The drawing under review shows one solid part. Ordinate dimensions are in mm from its lowest x, y, z. A direction names the side the tool comes from. Round coordinates to 2 decimals unless told otherwise and drop trailing zeros. Write each loop counter-clockwise with the first axis right and the second up, starting at its lowest first coordinate (ties: lowest second). Pieces come first, ordered by that corner, then holes. Notation, with made-up numbers: (30.25, -18.5) -> (34.25, -18.5) arc R18 ccw to (34.25, 3.5) -> close; hole circle Ø5 at (8.25, 47.25). An arc over 180 degrees is marked (long way). Answer in a Markdown table with one row per item.
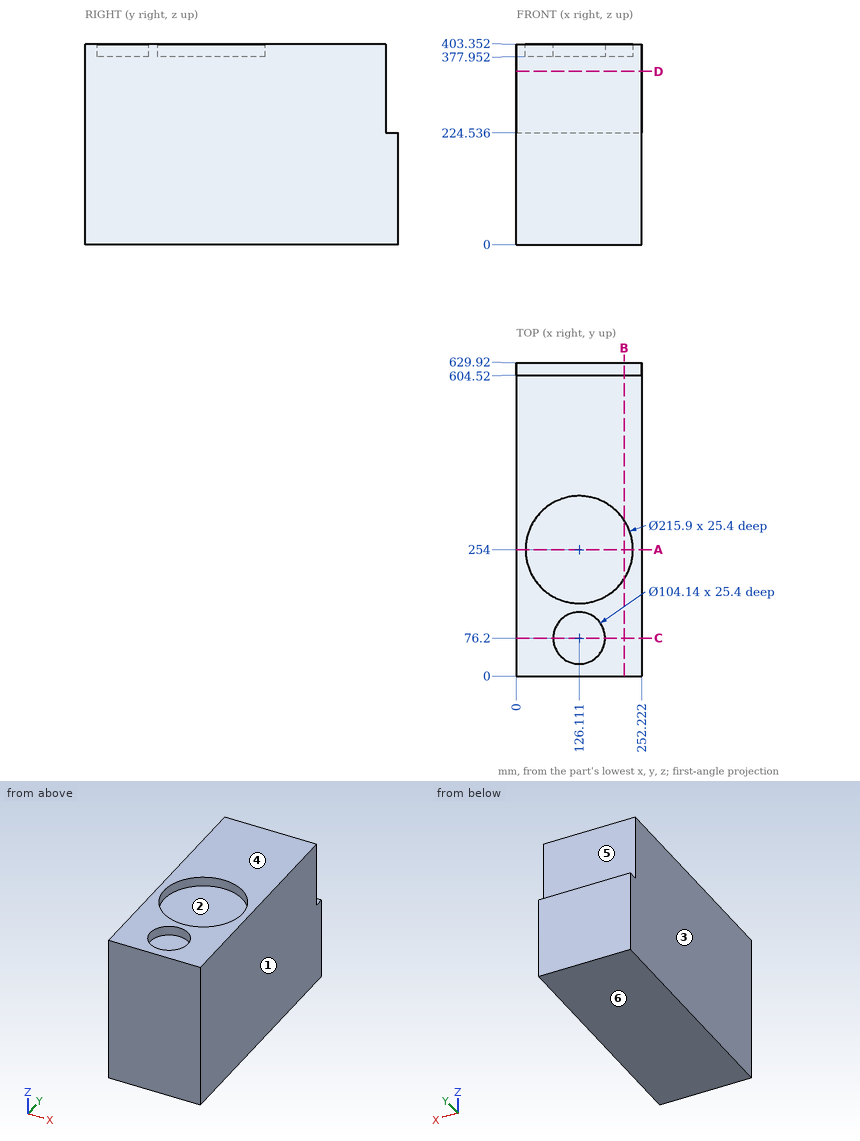
1) Consider section C-C on y = 76.2. State the section outline as (x, z) points, then the cut area to 3 significant figures.
Solved:
| item | result |
|---|---|
| outline | (0, 0) -> (252.22, 0) -> (252.22, 403.35) -> (178.18, 403.35) -> (178.18, 377.95) -> (74.04, 377.95) -> (74.04, 403.35) -> (0, 403.35) -> close |
| area | 99,100 mm² |
2) Consider section B-B on x = 216.5. State the section outline as (y, z) points, then the cut area to 3 significant figures.
Solved:
| item | result |
|---|---|
| outline | (0, 0) -> (629.92, 0) -> (629.92, 224.54) -> (604.52, 224.54) -> (604.52, 403.35) -> (313.02, 403.35) -> (313.02, 377.95) -> (194.98, 377.95) -> (194.98, 403.35) -> (0, 403.35) -> close |
| area | 247,000 mm² |
3) For the marked faces 5 and 6, list the 3-axis set-ups (+Z, -Z, +X, -X, +Y, -Y) from which the entire face can be reached by the end or side of a thin tool; tool diameter is ignored.
Solved:
| item | result |
|---|---|
| face 5 | +Z, +X, -X, +Y |
| face 6 | -Z, +X, -X, +Y, -Y |
4) Clearance check with flat-ended pins moving along their axes: pin 1 Ø1.5 at (x, y) = (111.5, 333) entering from +Z; pin 2 Ø10 at (x, z) = (146, 310) entering from +Y; pin 3 Ø12.5 at (x, y) = (127.5, 619) entering from +Z. State where each tip first meets the part, or that it passes through.
Solved:
| item | result |
|---|---|
| pin 1 | z = 377.95 |
| pin 2 | y = 604.52 |
| pin 3 | z = 224.54 |
5) For line 1 (X direction, y = 76, z = 389); line 2 (Z direction, x = 187, y = 171); line 3 (Y direction, x = 207, z = 375), list the stretches that pass through material, from the lowest coordinate up. Write a range as [from, to].
Solved:
| item | result |
|---|---|
| line 1 | [0, 74.04], [178.18, 252.22] |
| line 2 | [0, 377.95] |
| line 3 | [0, 604.52] |
6) Consider section D-D on z = 348.5. State the section outline as (x, y) points.
Solved:
| item | result |
|---|---|
| outline | (0, 0) -> (252.22, 0) -> (252.22, 604.52) -> (0, 604.52) -> close |
7) Mouldability with a two-part tool opening along X and no side actions: class the marked faces 1, 2, 3 and 4 as pulls with the +X half, pulls with the -X half, needs draft (parallel to the pull), parting line crosses it, or undercut.
Solved:
| item | result |
|---|---|
| face 1 | pulls with the +X half |
| face 2 | undercut |
| face 3 | pulls with the -X half |
| face 4 | needs draft |
8) Consider section A-A on y = 254. State the section outline as (x, z) points, then the cut area to 3 significant figures.
Solved:
| item | result |
|---|---|
| outline | (0, 0) -> (252.22, 0) -> (252.22, 403.35) -> (234.06, 403.35) -> (234.06, 377.95) -> (18.16, 377.95) -> (18.16, 403.35) -> (0, 403.35) -> close |
| area | 96,300 mm² |
